from build123d import *

# Parameters (mm, degrees)
BOSS_EXTRUDE1_DEPTH = 5
SKETCH3_W           = 119
SKETCH3_H           = 149
SKETCH3_W_2         = 113
SKETCH3_H_2         = 70
BOSS_EXTRUDE3_DEPTH = 30
SKETCH7_W           = 113
SKETCH7_H           = 3
CUT_EXTRUDE2_DEPTH  = 15
SKETCH8_R           = 5
CUT_EXTRUDE3_DEPTH  = 2
SKETCH9_R           = 2
CUT_EXTRUDE4_DEPTH  = 15


with BuildPart() as part:
    # Sketch2 → Boss-Extrude1 (new body)
    with BuildSketch(Plane(origin=(0, 0, 0), x_dir=(1, 0, 0), z_dir=(0, 1, 0))):
        Polygon((-66.5, 35), (-66.5, 38), (52.5, 38), (52.5, -111), (-66.5, -111), align=None)
    extrude(amount=BOSS_EXTRUDE1_DEPTH)

    # Sketch3 → Boss-Extrude3 (add)
    with BuildSketch(Plane(origin=(0, 5, 0), x_dir=(1, 0, 0), z_dir=(0, 1, 0))):
        with Locations((-7, -36.5)):
            Rectangle(SKETCH3_W, SKETCH3_H)
        with Locations((-7, 0)):
            Rectangle(SKETCH3_W_2, SKETCH3_H_2, mode=Mode.SUBTRACT)
        with Locations((-7, -73)):
            Rectangle(SKETCH3_W_2, SKETCH3_H_2, mode=Mode.SUBTRACT)
    extrude(amount=BOSS_EXTRUDE3_DEPTH)

    # Sketch7 → Cut-Extrude2 (cut)
    with BuildSketch(Plane(origin=(0, 35, 0), x_dir=(1, 0, 0), z_dir=(0, 1, 0))):
        with Locations((-7, -36.5)):
            Rectangle(SKETCH7_W, SKETCH7_H)
    extrude(amount=-CUT_EXTRUDE2_DEPTH, mode=Mode.SUBTRACT)

    # Sketch8 → Cut-Extrude3 (cut)
    with BuildSketch(Plane(origin=(0, 5, 0), x_dir=(1, 0, 0), z_dir=(0, 1, 0))):
        with Locations(Location((-55.5, 27, 0), (0, 0, 270))):
            Circle(SKETCH8_R)
        with Locations(Location((41.5, 27, 0), (0, 0, 90))):
            Circle(SKETCH8_R)
        with Locations(Location((41.5, -100, 0), (0, 0, 270))):
            Circle(SKETCH8_R)
        with Locations(Location((-55.5, -100, 0), (0, 0, 90))):
            Circle(SKETCH8_R)
    extrude(amount=-CUT_EXTRUDE3_DEPTH, mode=Mode.SUBTRACT)

    # Sketch9 → Cut-Extrude4 (cut)
    with BuildSketch(Plane(origin=(0, 3, 0), x_dir=(1, 0, 0), z_dir=(0, 1, 0))):
        with Locations(Location((41.5, 27, 0), (0, 0, 270))):
            Circle(SKETCH9_R)
        with Locations(Location((-55.5, 27, 0), (0, 0, 90))):
            Circle(SKETCH9_R)
        with Locations(Location((41.5, -100, 0), (0, 0, 90))):
            Circle(SKETCH9_R)
        with Locations(Location((-55.5, -100, 0), (0, 0, 270))):
            Circle(SKETCH9_R)
    extrude(amount=-CUT_EXTRUDE4_DEPTH, mode=Mode.SUBTRACT)


solid = part.part
Geometry: final body of the model. Coordinates: model frame, mm. A direction names the side the tool comes from. Round coordinates to 2 decimals unless told otherwise and drop trailing zeros. Loops run counter-clockwise (first coordinate to the right, second up) from the corner with the lowest first, then second, coordinate; pieces in that order, holes last. Notation, with made-up numbers: M 13.5,-10.75 L 70.5,-10.75 A7 cw 70.5,-1.75 Z; hole C -13,31.25 d10. An arc over 180 degrees is marked long. Put each result on its own line as item: value. Start each with the question number.
(1) Draft query along Z for faces 3 (the face through (-8, 20, 108)), 4 (the face through (-54.899, 1.521, 101.908)), 5 (the face through (-6, 0, 35)), 6 (the face through (-8, 17, -38)). Return one class per face: +Z half, -Z half, draft (parallel to the pull), parting line (faces both ways), or undercut.
(2) Section query A-A (x = 41.5). Return loops of the section in (y, z).
(3) Set-up query: faces 1 (the face through (38.121, 4.014, -23.315)), 2 (the face through (52.5, 17, 38)). Return all of +Z, -Z, +X, -X, +Y, -Y with unobstructed straight access to the full face (end or side cutting, diameter ignored); none if empty.
(4) Section query B-B (z = 100). Return loops of the section in (x, y).
(5) Material intervals for line 1 along X through (y, z) = (4, -27); line 2 along Z through (x, y) = (21, 10); line 3 along Z through (x, y) = (-55, 4), sorted ascending. Write a range as [from, to].
(6) Contact query for flat-ended pins moving along their axis: pin 1 Ø1.5 at (x, z) = (20.5, 36) entering from +Y; pin 2 Ø4 at (x, z) = (-43.5, 95) entering from +Y. Output: stop coordinate, or through.
(7) Section query D-D (x = 0). Return loops of the section in (y, z).
(8) Section query C-C (y = 7). Return loops of the section in (x, z).
Findings below:
1. face 3: undercut
1. face 4: undercut
1. face 5: draft
1. face 6: -Z half
2. outline: M 0,-38 L 35,-38 L 35,-35 L 5,-35 L 5,-32 L 3,-32 L 3,-29 L 0,-29 Z; M 0,-25 L 3,-25 L 3,-22 L 5,-22 L 5,35 L 20,35 L 20,38 L 5,38 L 5,95 L 3,95 L 3,98 L 0,98 Z; M 0,102 L 3,102 L 3,105 L 5,105 L 5,108 L 35,108 L 35,111 L 0,111 Z
3. face 1: +Y
3. face 2: +Z, -Z, +X, +Y, -Y
4. outline: M -66.5,0 L -57.5,0 L -57.5,3 L -60.5,3 L -60.5,5 L -63.5,5 L -63.5,35 L -66.5,35 Z; M -53.5,0 L 39.5,0 L 39.5,3 L 36.5,3 L 36.5,5 L -50.5,5 L -50.5,3 L -53.5,3 Z; M 43.5,0 L 52.5,0 L 52.5,35 L 49.5,35 L 49.5,5 L 46.5,5 L 46.5,3 L 43.5,3 Z
5. line 1: x = [-66.5, -60.5], [-50.5, 36.5], [46.5, 52.5]
5. line 2: z = [-38, -35], [35, 38], [108, 111]
5. line 3: z = [-38, -31.97], [-22.03, 95.03], [104.97, 111]
6. pin 1: stops at y = 20
6. pin 2: stops at y = 5
7. outline: M 0,-38 L 35,-38 L 35,-35 L 5,-35 L 5,35 L 20,35 L 20,38 L 5,38 L 5,108 L 35,108 L 35,111 L 0,111 Z
8. outline: M -66.5,-38 L 52.5,-38 L 52.5,111 L -66.5,111 Z; hole M -63.5,-35 L 49.5,-35 L 49.5,35 L -63.5,35 Z; hole M -63.5,38 L 49.5,38 L 49.5,108 L -63.5,108 Z
